```python
from build123d import *
from build123d.topology import SkipClean

# Parameters (mm, degrees)
SKETCH1_R           = 3.5
BOSS_EXTRUDE1_DEPTH = 5
SKETCH2_R           = 3
CUT_EXTRUDE1_DEPTH  = 4
SKETCH4_R           = 3.75
BOSS_EXTRUDE2_DEPTH = 2
SKETCH5_R           = 2.75
CUT_EXTRUDE2_DEPTH  = 1.8
SKETCH6_R           = 1.190625
CUT_EXTRUDE3_DEPTH  = 1.8
BOSS_EXTRUDE3_START = -1
BOSS_EXTRUDE3_DEPTH = 2
SKETCH9_R           = 0.9906
CUT_EXTRUDE4_DEPTH  = 20.055839
SKETCH10_R          = 0.396875
CUT_EXTRUDE5_DEPTH  = 20.055839


with BuildPart() as part:
    # Sketch1 → Boss-Extrude1 (new body)
    with BuildSketch(Plane(origin=(0, 0, 0), x_dir=(1, 0, 0), z_dir=(0, 1, 0))):
        with Locations(Location((0, 0, 0), (0, 0, 270))):
            Circle(SKETCH1_R)
    extrude(amount=BOSS_EXTRUDE1_DEPTH)

    # Sketch2 → Cut-Extrude1 (cut)
    with BuildSketch(Plane.XZ):
        with Locations(Location((0, 0, 0), (0, 0, 270))):
            Circle(SKETCH2_R)
    extrude(amount=-CUT_EXTRUDE1_DEPTH, mode=Mode.SUBTRACT)

    # Sketch4 → Boss-Extrude2 (add)
    with BuildSketch(Plane(origin=(0, 5, 0), x_dir=(1, 0, 0), z_dir=(0, 1, 0))):
        with Locations(Location((0, 0, 0), (0, 0, 270))):
            Circle(SKETCH4_R)
    extrude(amount=-BOSS_EXTRUDE2_DEPTH)

    # Sketch5 → Cut-Extrude2 (cut)
    with BuildSketch(Plane(origin=(0, 5, 0), x_dir=(1, 0, 0), z_dir=(0, 1, 0))):
        with Locations(Location((0, 0, 0), (0, 0, 270))):
            Circle(SKETCH5_R)
    extrude(amount=-CUT_EXTRUDE2_DEPTH, mode=Mode.SUBTRACT)

    # Sketch6 → Cut-Extrude3 (cut)
    with BuildSketch(Plane(origin=(0, 3.2, 0), x_dir=(1, 0, 0), z_dir=(0, 1, 0))):
        with Locations(Location((0, 0, 0), (0, 0, 270))):
            Circle(SKETCH6_R)
    extrude(amount=-CUT_EXTRUDE3_DEPTH, mode=Mode.SUBTRACT)

    # Sketch8 → Boss-Extrude3 (add)
    with SkipClean():  # the faces are left unmerged after this step: merging them gives an invalid solid
        with BuildSketch(Plane.XZ.offset(-3).offset(BOSS_EXTRUDE3_START)):
            with BuildLine():
                Line((0, 3.75), (-16.802200952, 1.675319737))
                ThreePointArc((-16.802200952, 1.675319737), (-17.83614958, 1.130657807), (-18.25, 0.037756066))
                Line((-18.25, 0.037756066), (-18.25, -0.037756066))
                ThreePointArc((-18.25, -0.037756066), (-17.83614958, -1.130657807), (-16.802200952, -1.675319737))
                Line((-16.802200952, -1.675319737), (0, -3.75))
                ThreePointArc((0, -3.75), (3.75, 0), (0, 3.75))
            make_face()
        boss_extrude3 = extrude(amount=BOSS_EXTRUDE3_DEPTH)

    # Mirror1: Boss-Extrude3 across plane
    with SkipClean():  # the faces are left unmerged after this step: merging them gives an invalid solid
        add(boss_extrude3.mirror(Plane(origin=(0, 0, 0), x_dir=(0, 0, 1), z_dir=(1, 0, 0))))
    add(part.part.scale(1), mode=Mode.REPLACE)  # the faces are merged on a copy

    # Sketch9 → Cut-Extrude4 (cut, through all)
    with BuildSketch(Plane(origin=(0, 4, 0), x_dir=(1, 0, 0), z_dir=(0, 1, 0))):
        with Locations(Location((0, 0, 0), (0, 0, 270))):
            Circle(SKETCH9_R)
    extrude(amount=-CUT_EXTRUDE4_DEPTH, mode=Mode.SUBTRACT)

    # Sketch10 → Cut-Extrude5 (cut, through all)
    with BuildSketch(Plane(origin=(0, 4, 0), x_dir=(1, 0, 0), z_dir=(0, 1, 0))):
        with Locations(Location((-11.509375, 0, 0), (0, 0, 270))):
            Circle(SKETCH10_R)
    cut_extrude5 = extrude(amount=-CUT_EXTRUDE5_DEPTH, mode=Mode.SUBTRACT)

    # Mirror2: Cut-Extrude5 across plane
    add(cut_extrude5.mirror(Plane(origin=(0, 0, 0), x_dir=(0, 0, 1), z_dir=(1, 0, 0))), mode=Mode.SUBTRACT)


solid = part.part
```
Geometry: final body of the model. Coordinates: model frame, mm. A direction names the side the tool comes from. Coordinates: 2 decimals unless noted, no trailing zeros. Loops run counter-clockwise (first coordinate to the right, second up) from the corner with the lowest first, then second, coordinate; pieces in that order, holes last. Notation, with made-up numbers: (-11, 78.5) -> (34, 78.5) arc R25 ccw to (34, 96.5) -> close; hole circle Ø1 at (-36.5, 27). An arc over 180 degrees is marked (long way). Use a Markdown table: item, result. Add a question column.
(1) Line query: line 1 along X through (y, z) = (3.3, 0); line 2 along Y through (x, z) = (10, -0.75); line 3 along X through (y, z) = (1, -1). Output: solid intervals per line, ascending.
(2) Section query D-D, the plane x = 9. Return loops of the section in (y, z), plus the area to 3 significant figures.
(3) Section query C-C, the plane x = -8. Return loops of the section in (y, z).
(4) Section query B-B, the plane x = -2. Return loops of the section in (y, z), plus the area to 3 significant figures.
(5) Access query for faces 4 (the flat face through (-1, 2, 1)), 5 (the flat face through (1.2, 4, 0)), 6 (the flat face through (-8.968, 3.014, -2.643)). Directions: +Z, -Z, +X, -X, +Y, -Y. A direction counts if a zero-diameter tool reaches every point of the face in a straight line with its end or side. Return the directions, or none.
(6) Section query A-A, the plane y = 0.75. Return loops of the section in (x, z).
(7) Pin query (flat end, axial travel): pin 1 Ø1.5 at (x, z) = (8, 2.5) entering from +Y; pin 2 Ø2 at (x, z) = (8, -1) entering from -Y; pin 3 Ø1.5 at (x, y) = (-12.5, 3) entering from -Z. Return the tip coordinate at first contact, or that it passes through.
(8) Mould query, pull axis X, two halves, no side actions, for faces 1 (the flat face through (-10, 4, 0)), 2 (the cylindrical face through (0.9, 0.99, -2.86)), 3 (the cylindrical face through (17.847, 3.014, -1.118)). Classes: pulls with the +X half, pulls with the -X half, needs draft (parallel to the pull), parting line crosses it, or undercut.
Answer:
| question | item | result |
|---|---|---|
| 1 | line 1 | x = -18.25 to -11.91, -11.11 to -0.99, 0.99 to 11.11, 11.91 to 18.25 |
| 1 | line 2 | y = 2 to 4 |
| 1 | line 3 | x = -3.35 to -2.83, 2.83 to 3.35 |
| 2 | outline | (2, -2.64) -> (4, -2.64) -> (4, 2.64) -> (2, 2.64) -> close |
| 2 | area | 10.6 mm^2 |
| 3 | outline | (2, -2.76) -> (4, -2.76) -> (4, 2.76) -> (2, 2.76) -> close |
| 4 | outline | (0, -2.87) -> (2, -2.87) -> (2, -3.5) -> (4, -3.5) -> (4, -3.17) -> (5, -3.17) -> (5, -1.89) -> (4, -1.89) -> (4, 1.89) -> (5, 1.89) -> (5, 3.17) -> (4, 3.17) -> (4, 3.5) -> (2, 3.5) -> (2, 2.87) -> (0, 2.87) -> (0, 2.24) -> (2, 2.24) -> (2, -2.24) -> (0, -2.24) -> close |
| 4 | area | 19.1 mm^2 |
| 5 | face 4 | -Y |
| 5 | face 5 | +Y |
| 5 | face 6 | -Z, -X, +Y, -Y |
| 6 | outline | circle Ø7 at (0, 0); hole circle Ø6 at (0, 0) |
| 7 | pin 1 | stops at y = 4 |
| 7 | pin 2 | stops at y = 2 |
| 7 | pin 3 | stops at z = -2.3 |
| 8 | face 1 | needs draft |
| 8 | face 2 | undercut |
| 8 | face 3 | pulls with the +X half |
